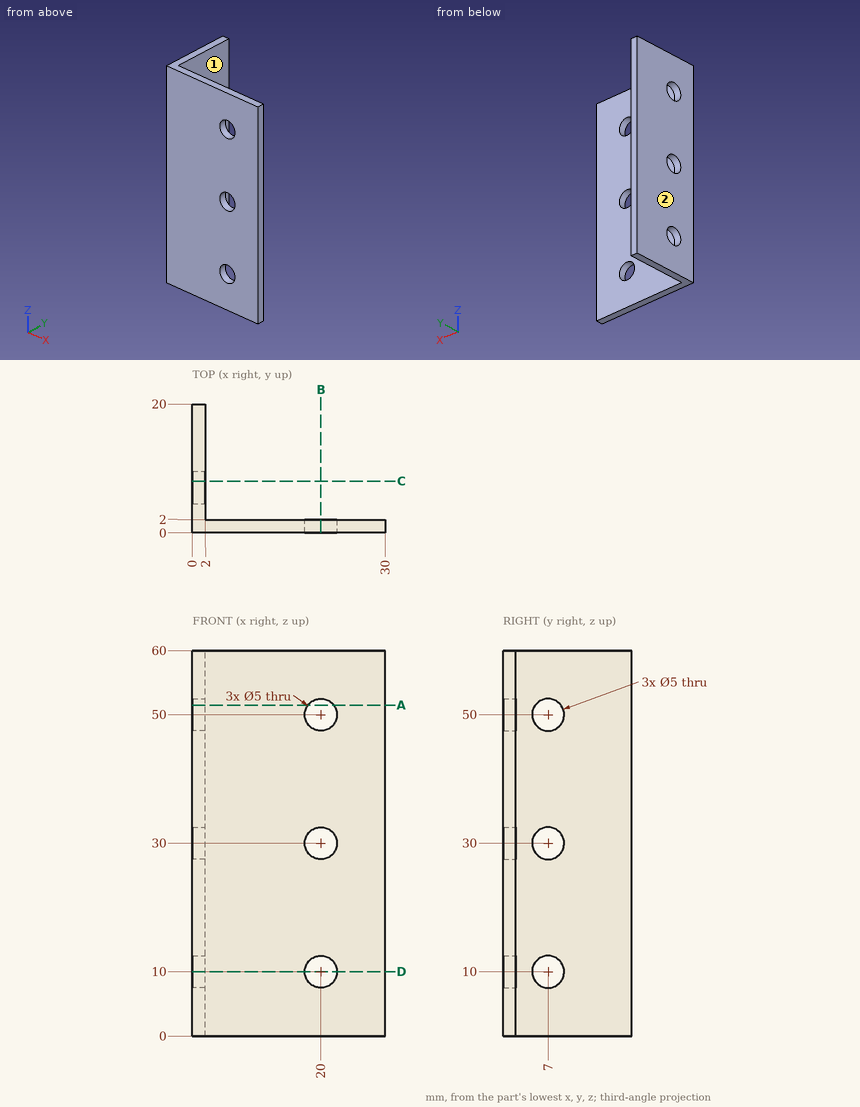
The figure shows three views and two pictorial views of one solid part (mm, origin at its lowest corner). Answer the questions. A direction names the side the tool comes from. Give positions to 0.01 mm unless a question says otherwise; leave off trailing zeros. Loops run counter-clockwise (first coordinate to the right, second up) from the corner with the lowest first, then second, coordinate; pieces in that order, holes last. Notation, with made-up numbers: (-11.75, 82) -> (32.25, 82) arc R29 ccw to (32.25, 113) -> close; hole circle Ø4 at (89, 86). An arc over 180 degrees is marked (long way). Use a Markdown table: item, result. Add a question column.
1. Section A-A on z = 51.5 is taken. Determine the outline of the cut face in (x, y).
2. Section B-B on x = 20 is taken. Determine the outline of the cut face in (y, z).
3. Section D-D on z = 10 is taken. Determine the outline of the cut face in (x, y), and give its area (3 significant figures).
4. For the marked faces 1 and 2, determine the directions among +Z, -Z, +X, -X, +Y, -Y from which every point of the face is accessible in a straight line to the end or side of a thin tool.
5. Section C-C on y = 8 is taken. Determine the outline of the cut face in (x, z).
6. Flat-ended cylindrical pins translate along their axes: pin 1 Ø5 at (y, z) = (11, 40.5) entering from -X; pin 2 Ø8.5 at (x, z) = (14.5, 30) entering from +Y; pin 3 Ø4 at (x, z) = (20, 10) entering from -Y; pin 4 Ø6.5 at (y, z) = (7, 10) entering from +X. Find the tip coordinate at first contact, or state that the pin passes through.
7. Find the intervals of material crossed by probe 1 along Z at (x, y) = (20, 1.5); probe 2 along X at (y, z) = (1.2, 50); probe 3 along Y at (x, z) = (0.85, 50), in increasing order.
Results below:
| question | item | result |
|---|---|---|
| 1 | outline | (0, 0) -> (18, 0) -> (18, 2) -> (2, 2) -> (2, 5) -> (0, 5) -> close; (0, 9) -> (2, 9) -> (2, 20) -> (0, 20) -> close; (22, 0) -> (30, 0) -> (30, 2) -> (22, 2) -> close |
| 2 | outline | (0, 0) -> (2, 0) -> (2, 7.5) -> (0, 7.5) -> close; (0, 12.5) -> (2, 12.5) -> (2, 27.5) -> (0, 27.5) -> close; (0, 32.5) -> (2, 32.5) -> (2, 47.5) -> (0, 47.5) -> close; (0, 52.5) -> (2, 52.5) -> (2, 60) -> (0, 60) -> close |
| 3 | outline | (0, 0) -> (17.5, 0) -> (17.5, 2) -> (2, 2) -> (2, 4.5) -> (0, 4.5) -> close; (0, 9.5) -> (2, 9.5) -> (2, 20) -> (0, 20) -> close; (22.5, 0) -> (30, 0) -> (30, 2) -> (22.5, 2) -> close |
| 3 | area | 76.0 mm^2 |
| 4 | face 1 | +Z, -Z, +X, +Y |
| 4 | face 2 | +Z, -Z, -X, +Y, -Y |
| 5 | outline | (0, 0) -> (2, 0) -> (2, 7.71) -> (0, 7.71) -> close; (0, 12.29) -> (2, 12.29) -> (2, 27.71) -> (0, 27.71) -> close; (0, 32.29) -> (2, 32.29) -> (2, 47.71) -> (0, 47.71) -> close; (0, 52.29) -> (2, 52.29) -> (2, 60) -> (0, 60) -> close |
| 6 | pin 1 | stops at x = 0 |
| 6 | pin 2 | stops at y = 2 |
| 6 | pin 3 | passes through |
| 6 | pin 4 | stops at x = 2 |
| 7 | probe 1 | z = 0 to 7.5, 12.5 to 27.5, 32.5 to 47.5, 52.5 to 60 |
| 7 | probe 2 | x = 0 to 17.5, 22.5 to 30 |
| 7 | probe 3 | y = 0 to 4.5, 9.5 to 20 |
